Read the model definition and answer for the solid it produces. Units are mm, in the model's axes. A direction names the side the tool comes from. Coordinates: 2 decimals unless noted, no trailing zeros. Write each loop counter-clockwise with the first axis right and the second up, starting at its lowest first coordinate (ties: lowest second). Pieces come first, ordered by that corner, then holes. Notation, with made-up numbers: M 36,-38 L 50,-38 A21 ccw 50,-2 Z; hole C 85,80 d9. An arc over 180 degrees is marked long. Write item = value, one per line.
from build123d import *
from build123d.topology import SkipClean

# Parameters (mm, degrees)
BOSS_EXTRUDE1_DEPTH             = 25
BOSS_EXTRUDE2_REACH             = 65.362
BOSS_EXTRUDE2_DIRECTION_2_DEPTH = 30
SKETCH9_R                       = 2.05
CUT_EXTRUDE3_DEPTH              = 35
BOSS_EXTRUDE5_REACH             = 63.601
SKETCH13_R                      = 1.55
CUT_EXTRUDE4_DEPTH              = 88.693844753
SKETCH16_W                      = 63
SKETCH16_H                      = 45
CUT_EXTRUDE5_DEPTH              = 65.196143
BOSS_EXTRUDE6_DEPTH             = 17.5
SKETCH18_R                      = 2.05
CUT_EXTRUDE6_DEPTH              = 17.5
CUT_EXTRUDE7_START              = -7.35
CUT_EXTRUDE7_DEPTH              = 3.3


with BuildPart() as part:
    # Sketch1 → Boss-Extrude1 (new, symmetric)
    with BuildSketch(Plane.XY):
        with BuildLine():
            Line((-17.5, 22.5), (-17.5, 0))
            Line((-17.5, 0), (17.5, 0))
            Line((17.5, 0), (17.5, 22.5))
            Line((17.5, 22.5), (12.5, 22.5))
            ThreePointArc((12.5, 22.5), (0, 10), (-12.5, 22.5))
            Line((-12.5, 22.5), (-17.5, 22.5))
        make_face()
    boss_extrude1 = extrude(amount=BOSS_EXTRUDE1_DEPTH, both=True)

    # Boss-Extrude2: up to this face of the body (flat: up to its plane)
    boss_extrude2_end = Plane(part.part.faces().sort_by_distance((17.5, 11.25, 0))[0])
    # Sketch5 → Boss-Extrude2 (add, up to the picked face)
    with BuildSketch(Plane(origin=(26.115381057, 0, 15.077722283), x_dir=(0.500000000000001, 0, -0.8660254037844382), z_dir=(0.8660254037844382, 0, 0.500000000000001)), mode=Mode.PRIVATE) as boss_extrude2_sk1:
        with BuildLine():
            Line((-8.7, 22.5), (-3.75, 22.5))
            ThreePointArc((-3.75, 22.5), (8.75, 10), (21.25, 22.5))
            Line((21.25, 22.5), (26.2, 22.5))
            ThreePointArc((26.2, 22.5), (8.75, 5.05), (-8.7, 22.5))
        make_face()
    boss_extrude2_tool1 = split(extrude(boss_extrude2_sk1.sketch, amount=-BOSS_EXTRUDE2_REACH, mode=Mode.PRIVATE), bisect_by=boss_extrude2_end, keep=Keep.BOTH, mode=Mode.PRIVATE)
    boss_extrude2 = boss_extrude2_tool1.solids().sort_by(Axis((23.002881, 22.109806, 20.46873), (-0.8660254037844382, 0, -0.500000000000001)))[0]
    add(boss_extrude2)

    # Sketch5 → Boss-Extrude2 direction 2 (add)
    with BuildSketch(Plane(origin=(26.115381057, 0, 15.077722283), x_dir=(0.500000000000001, 0, -0.8660254037844382), z_dir=(0.8660254037844382, 0, 0.500000000000001))):
        with BuildLine():
            Line((-8.7, 22.5), (-3.75, 22.5))
            ThreePointArc((-3.75, 22.5), (8.75, 10), (21.25, 22.5))
            Line((21.25, 22.5), (26.2, 22.5))
            ThreePointArc((26.2, 22.5), (8.75, 5.05), (-8.7, 22.5))
        make_face()
    boss_extrude2_direction_2 = extrude(amount=BOSS_EXTRUDE2_DIRECTION_2_DEPTH)

    # Sketch9 → Cut-Extrude3 (cut)
    with BuildSketch(Plane.ZY.offset(17.5)):
        with Locations((-18, 5)):
            Circle(SKETCH9_R)
    cut_extrude3 = extrude(amount=-CUT_EXTRUDE3_DEPTH, mode=Mode.SUBTRACT)

    # Boss-Extrude5: up to this face of the body (flat: up to its plane)
    boss_extrude5_end = Plane(part.part.faces().sort_by_distance((17.5, 17.19483523, 0))[0])
    # Sketch12 → Boss-Extrude5 (add, up to the picked face)
    with BuildSketch(Plane(origin=(21.973076211, 0, 12.686161466), x_dir=(0.4999999999999999, 0, -0.8660254037844388), z_dir=(0.8660254037844388, 0, 0.4999999999999999)), mode=Mode.PRIVATE) as boss_extrude5_sk1:
        with BuildLine():
            Line((-3.75, 22.5), (21.25, 22.5))
            ThreePointArc((21.25, 22.5), (8.75, 10), (-3.75, 22.5))
        make_face()
    boss_extrude5_tool1 = split(extrude(boss_extrude5_sk1.sketch, amount=-BOSS_EXTRUDE5_REACH, mode=Mode.PRIVATE), bisect_by=boss_extrude5_end, keep=Keep.BOTH, mode=Mode.PRIVATE)
    boss_extrude5 = boss_extrude5_tool1.solids().sort_by(Axis((26.348076, 17.194835, 5.108439), (-0.8660254037844388, 0, -0.4999999999999999)))[0]
    add(boss_extrude5)

    # Mirror1: Boss-Extrude1, Boss-Extrude2, Boss-Extrude2 direction 2, Cut-Extrude3, Boss-Extrude5 across plane
    with SkipClean():  # the faces are left unmerged after this step: merging them gives an invalid solid
        add(boss_extrude1.mirror(Plane(origin=(17.5, 22.5, 25), x_dir=(0, 0, 1), z_dir=(0, -1, 0))))
        add(boss_extrude2.mirror(Plane(origin=(17.5, 22.5, 25), x_dir=(0, 0, 1), z_dir=(0, -1, 0))))
        add(boss_extrude2_direction_2.mirror(Plane(origin=(17.5, 22.5, 25), x_dir=(0, 0, 1), z_dir=(0, -1, 0))))
        add(cut_extrude3.mirror(Plane(origin=(17.5, 22.5, 25), x_dir=(0, 0, 1), z_dir=(0, -1, 0))), mode=Mode.SUBTRACT)
        add(boss_extrude5.mirror(Plane(origin=(17.5, 22.5, 25), x_dir=(0, 0, 1), z_dir=(0, -1, 0))))

    # Sketch13 → Cut-Extrude4 (cut, through all)
    with SkipClean():  # the faces are left unmerged after this step: merging them gives an invalid solid
        with BuildSketch(Plane(origin=(0, 0, 0), x_dir=(1, 0, 0), z_dir=(0, 1, 0))):
            with Locations(Location((43.480762114, -15, 0), (0, 0, 90))):
                Circle(SKETCH13_R)
        extrude(amount=CUT_EXTRUDE4_DEPTH, mode=Mode.SUBTRACT)

    # Sketch16 → Cut-Extrude5 (cut)
    with BuildSketch(Plane(origin=(0, 0, 0), x_dir=(0, 0, -1), z_dir=(1, 0, 0))):
        with Locations((-6.5, 22.5)):
            Rectangle(SKETCH16_W, SKETCH16_H)
    extrude(amount=CUT_EXTRUDE5_DEPTH, mode=Mode.SUBTRACT)

    # Sketch17 → Boss-Extrude6 (add)
    with BuildSketch(Plane.ZY.offset(17.5)):
        with BuildLine():
            Line((13, 0), (23, 0))
            ThreePointArc((23, 0), (18, -5), (13, 0))
        make_face()
    boss_extrude6 = extrude(amount=-BOSS_EXTRUDE6_DEPTH)

    # Sketch18 → Cut-Extrude6 (cut)
    with BuildSketch(Plane.ZY.offset(17.5)):
        with Locations(Location((18, 0, 0), (0, 0, 270))):
            Circle(SKETCH18_R)
    cut_extrude6 = extrude(amount=-CUT_EXTRUDE6_DEPTH, mode=Mode.SUBTRACT)

    # Mirror2: Boss-Extrude6, Cut-Extrude6 across plane
    add(boss_extrude6.mirror(Plane.ZX.offset(22.5)))
    add(cut_extrude6.mirror(Plane.ZX.offset(22.5)), mode=Mode.SUBTRACT)

    # Sketch20 → Cut-Extrude7 (cut)
    with BuildSketch(Plane(origin=(0, 0, 0), x_dir=(0, 0, -1), z_dir=(1, 0, 0)).offset(CUT_EXTRUDE7_START)):
        Polygon((22.156921938, 40), (20.078460969, 43.6), (15.921539031, 43.6), (13.843078062, 40), (15.921539031, 36.4), (20.078460969, 36.4), align=None)
        Polygon((-13.843078062, 0), (-15.921539031, 3.6), (-20.078460969, 3.6), (-22.156921938, 0), (-20.078460969, -3.6), (-15.921539031, -3.6), align=None)
    extrude(amount=-CUT_EXTRUDE7_DEPTH, mode=Mode.SUBTRACT)


solid = part.part
Item 1: Find section D-D (z = -18). Determine the outline of the cut face in (x, y).
Worked answers:
outline = M -17.5,0 L 0,0 L 0,2.95 L -17.5,2.95 Z; M -17.5,7.05 L 0,7.05 L 0,10 A12.5 cw 0,35 L 0,37.95 L -7.35,37.95 L -7.35,36.4 L -10.65,36.4 L -10.65,37.95 L -17.5,37.95 Z; M -17.5,42.05 L -10.65,42.05 L -10.65,43.6 L -7.35,43.6 L -7.35,42.05 L 0,42.05 L 0,45 L -17.5,45 Z
Item 2: Consider line 1 along Y through (x, z) = (-16.5, -18); line 2 along X through (y, z) = (40, -21.5); line 3 along Y through (x, z) = (-16, -19.5). Determine where each line is inside the solid, lowest interval first. Write a range as from..to.
Worked answers:
line_1 = 0..2.95, 7.05..37.95, 42.05..45
line_2 = -17.5..-10.65, -7.35..0
line_3 = 0..3.6, 6.4..38.6, 41.4..45
Item 3: Find section C-C (x = -15.25). Determine the outline of the cut face in (y, z).
Worked answers:
outline = M 0,-25 L 45,-25 L 45,13 A5 ccw 45,23 L 45,25 L 0,25 L 0,23 A5 ccw 0,13 Z; hole C 0,18 d4.1; hole C 5,-18 d4.1; hole C 40,-18 d4.1; hole C 45,18 d4.1
Item 4: Find section A-A (x = -2). Determine the outline of the cut face in (y, z), and give its area (3 significant figures).
Worked answers:
outline = M 0,-25 L 10.16,-25 L 10.16,25 L 0,25 L 0,23 A5 ccw 0,13 Z; M 34.84,-25 L 45,-25 L 45,13 A5 ccw 45,23 L 45,25 L 34.84,25 Z; hole C 0,18 d4.1; hole C 5,-18 d4.1; hole C 40,-18 d4.1; hole C 45,18 d4.1
area = 1,040 mm²
Item 5: Flat-ended cylindrical pins translate along their axes: pin 1 (9 mm diameter, centred on x = -10.5, z = 2.5, fed in from -Y); pin 2 (10 mm diameter, centred on x = -10, z = 2, fed in from +Y); pin 3 (1 mm diameter, centred on y = 27.5, z = -19.5, fed in from +X) (3 decimals). Find the tip coordinate at first contact, or state that the pin passes through.
Worked answers:
pin_1 = 0
pin_2 = 45
pin_3 = -11.225
Item 6: Which of the six approach directions +Z, -Z, +X, -X, +Y, -Y give full straight-line access (tool end or side, diameter ignored) to faces 4 (the face through (-9, 2, 21)), 5 (the face through (-9, -5, 18)), 6 (the face through (-3.7, 1.5, 19.4)), 7 (the face through (-9, 0, 24)), 8 (the face through (-9, 45, 24))?
Worked answers:
face_4 = none
face_5 = +X, -X, -Y
face_6 = +X, -X
face_7 = +Z, +X, -X, -Y
face_8 = +Z, +X, -X, +Y
Item 7: Find section B-B (z = 18). Determine the outline of the cut face in (x, y), and give its area (3 significant figures).
Worked answers:
outline = M -17.5,-5 L 0,-5 L 0,-2.05 L -7.35,-2.05 L -7.35,-3.6 L -10.65,-3.6 L -10.65,-2.05 L -17.5,-2.05 Z; M -17.5,2.05 L -10.65,2.05 L -10.65,3.6 L -7.35,3.6 L -7.35,2.05 L 0,2.05 L 0,10 A12.5 cw 0,35 L 0,42.95 L -17.5,42.95 Z; M -17.5,47.05 L 0,47.05 L 0,50 L -17.5,50 Z
area = 563 mm²
Item 8: For a pull along X with two mould halves and no side action, classify faces 1 (the face through (-9, 38, -21)), 2 (the face through (-3.726, 37.967, -18.267)), 3 (the face through (0, 41, 0)) as released by +X, released by -X, zero draft, split by the parting line, or undercut.
Worked answers:
face_1 = undercut
face_2 = zero draft
face_3 = released by +X
